Geometry check sheet. Reference: drawing and pictorial views, mm from the part's lowest x, y, z. A direction names the side the tool comes from. Round coordinates to 2 decimals unless told otherwise and drop trailing zeros. Loops run counter-clockwise (first coordinate to the right, second up) from the corner with the lowest first, then second, coordinate; pieces in that order, holes last. Notation, with made-up numbers: (76.5, -4.5) -> (89.5, -4.5) arc R31 cw to (89.5, 27.5) -> close; hole circle Ø11 at (82.25, 72). An arc over 180 degrees is marked (long way). Write item = value, one per line.
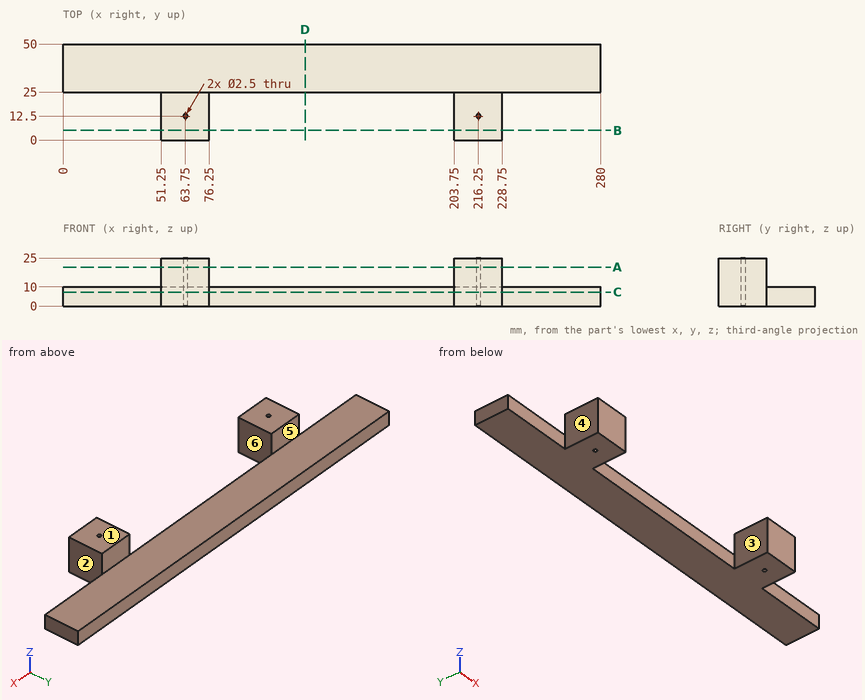
(1) Set-up check for the marked faces 4, 5 and 6: record each of +Z, -Z, +X, -X, +Y, -Y from which the full face is reachable in a straight line by a thin tool's end or side.
Filled sheet:
face_4 = +Z, -Z, -X, -Y
face_5 = +Z, +X, -X, +Y
face_6 = +Z, -Z, -Y
(2) Material ranges on probe 1 along Y at (x, z) = (216.25, 16); probe 2 along Y at (x, z) = (216.25, 7.5); probe 3 along X at (y, z) = (5, 12.5), recorded low to high. Write a range as from..to.
Filled sheet:
probe_1 = 0..11.25, 13.75..25
probe_2 = 0..11.25, 13.75..50
probe_3 = 51.25..76.25, 203.75..228.75
(3) Draft check along X on the marked faces 1, 2 and 3. Enter one of: released by +X, released by -X, zero draft, split by the parting line, or undercut.
Filled sheet:
face_1 = zero draft
face_2 = released by +X
face_3 = undercut
(4) Sectioned sample at D-D, the plane x = 126. Record the cut outline in (y, z), and give its area (3 significant figures).
Filled sheet:
outline = (25, 0) -> (50, 0) -> (50, 10) -> (25, 10) -> close
area = 250 mm2
(5) Sectioned sample at C-C, the plane z = 7.25. Record the cut outline in (x, y).
Filled sheet:
outline = (0, 25) -> (51.25, 25) -> (51.25, 0) -> (76.25, 0) -> (76.25, 25) -> (203.75, 25) -> (203.75, 0) -> (228.75, 0) -> (228.75, 25) -> (280, 25) -> (280, 50) -> (0, 50) -> close; hole circle Ø2.5 at (63.75, 12.5); hole circle Ø2.5 at (216.25, 12.5)
(6) Sectioned sample at B-B, the plane y = 5. Record the cut outline in (x, z), and give its area (3 significant figures).
Filled sheet:
outline = (51.25, 0) -> (76.25, 0) -> (76.25, 25) -> (51.25, 25) -> close; (203.75, 0) -> (228.75, 0) -> (228.75, 25) -> (203.75, 25) -> close
area = 1,250 mm2
(7) Sectioned sample at A-A, the plane z = 20.25. Record the cut outline in (x, y).
Filled sheet:
outline = (51.25, 0) -> (76.25, 0) -> (76.25, 25) -> (51.25, 25) -> close; (203.75, 0) -> (228.75, 0) -> (228.75, 25) -> (203.75, 25) -> close; hole circle Ø2.5 at (63.75, 12.5); hole circle Ø2.5 at (216.25, 12.5)
(8) Go/stop test with flat-tipped pins: pin 1 Ø3 at (y, z) = (22.5, 3.5) entering from -X; pin 2 Ø4.5 at (x, z) = (67, 14.5) entering from +Y; pin 3 Ø20 at (x, y) = (87, 32.5) entering from +Z. Record where each tip stops, or that it passes through.
Filled sheet:
pin_1 = 51.25
pin_2 = 25
pin_3 = 10
